Input: part model. Units: mm. Frame: model coordinates. A direction names the side the tool comes from. Coordinates: 2 decimals unless noted, no trailing zeros. Order: outer loops, then holes, each group sorted by start corner. A loop starts at its lowest first (then second) coordinate and runs counter-clockwise, first axis right, second up.
from build123d import *

# Parameters (mm, degrees)
F1_DEPTH     = 30
F2_R         = 14.99999
F4_DEPTH     = 219.001
F5_T1_DEPTH  = 2e-05
F5_T6_ANGLE  = 163.702935025
F5_T12_ANGLE = 163.702935025
F5_T18_ANGLE = 163.702935025
F5_T24_ANGLE = 163.702935025
F6_SIZE      = 5
F7_R         = 2.5
F8_DEPTH     = 139.001
F9_W         = 20
F9_H         = 20
F11_R        = 2.5
F12_DEPTH    = 20.001
F13_SIZE     = 2.5
F14_W        = 5
F14_H        = 25
F15_DEPTH    = 30
F16_R        = 14.99999
F17_R        = 5
F18_DEPTH    = 7.5
F19_SIZE     = 2.49999


# Not quite as in the source:
# - a fillet or chamfer that OpenCascade refuses, or shapes differently, is made with other operations: its cross-section is extruded or revolved along the edge and cut away or added
# - a fillet or chamfer is up to 0.001 mm smaller than in the source, because OpenCascade refuses the exact size


with BuildPart() as f1:
    # F0 (on Front) → F1 (new body)
    with BuildSketch(Plane.XZ):
        Polygon((-109.5, 0), (0, 0), (109.5, 0), (109.5, 20), (29.5, 20), (29.5, 50), (19.5, 50), (19.5, 20), (0, 20), (-19.5, 20), (-19.5, 50), (-29.5, 50), (-29.5, 20), (-109.5, 20), align=None)
    extrude(amount=F1_DEPTH)

    # F2 (radius 15 in the source; OpenCascade refuses exactly that, so slightly less here)
    f2_edges = [f1.edges().sort_by_distance(p)[0] for p in [
        (-69.5, 0, 20),
        (-69.5, -30, 20),
        (69.5, 0, 20),
        (69.5, -30, 20),
    ]]
    fillet(f2_edges, radius=F2_R)

    # F3 (on face) → F4 (cut, through all)
    with BuildSketch(Plane(origin=(-109.5, 0, 0), x_dir=(0, -1, 0), z_dir=(-1, 0, 0))):
        with BuildLine():
            Line((25, 0), (25, 5))
            ThreePointArc((25, 5), (15, 15), (5, 5))
            Line((5, 5), (5, 0))
            Line((5, 0), (25, 0))
        make_face()
    extrude(amount=-F4_DEPTH, mode=Mode.SUBTRACT)

    # F5: chamfer of 7.5 on 4 edges, made by hand

    # F5_s2 → F5_t1 (join)
    with BuildSketch(Plane.XZ.offset(14.99999)):
        Polygon((-37, 20), (-29.5, 27.5), (-29.5, 20), align=None)
        Polygon((37, 20), (29.5, 27.5), (29.5, 20), align=None)
    extrude(amount=F5_T1_DEPTH)


with BuildPart() as f5_tool4:
    # F5_s5 → F5_t6 (revolve)
    with BuildSketch(Plane(origin=(0, -12.4720838446, -3.6463990318), x_dir=(1, 0, 0), z_dir=(0, -0.9598196681, -0.2806175417))):
        Polygon((-37, -5.9916217418), (-29.5, -13.4916217418), (-29.5, -5.9916217418), align=None)
    revolve(axis=Axis((-29.5, -14.99999, 5.00001), (1, 0, 0)), revolution_arc=F5_T6_ANGLE)

    split(bisect_by=Plane.XZ, keep=Keep.TOP)

    split(bisect_by=Plane.XY, keep=Keep.TOP)


with BuildPart() as f1_1:
    add(f1.part)

    # F5_t3: union F5_tool4
    add(f5_tool4.part)


with BuildPart() as f5_tool10:
    # F5_s11 → F5_t12 (revolve)
    with BuildSketch(Plane(origin=(0, -12.4720838446, -3.6463990318), x_dir=(1, 0, 0), z_dir=(0, -0.9598196681, -0.2806175417))):
        Polygon((29.5, -13.4916217418), (37, -5.9916217418), (29.5, -5.9916217418), align=None)
    revolve(axis=Axis((29.5, -14.99999, 5.00001), (1, 0, 0)), revolution_arc=F5_T12_ANGLE)

    split(bisect_by=Plane.XZ, keep=Keep.TOP)

    split(bisect_by=Plane.XY, keep=Keep.TOP)


with BuildPart() as f1_2:
    add(f1_1.part)

    # F5_t9: union F5_tool10
    add(f5_tool10.part)


with BuildPart() as f5_tool16:
    # F5_s17 → F5_t18 (revolve)
    with BuildSketch(Plane.XZ.offset(15.00001)):
        Polygon((37, 20), (29.5, 27.5), (29.5, 20), align=None)
    revolve(axis=Axis((29.5, -15.00001, 5.00001), (1, 0, 0)), revolution_arc=F5_T18_ANGLE)

    split(bisect_by=Plane.XY, keep=Keep.TOP)

    split(bisect_by=Plane.XZ.offset(30), keep=Keep.BOTTOM)


with BuildPart() as f1_3:
    add(f1_2.part)

    # F5_t15: union F5_tool16
    add(f5_tool16.part)


with BuildPart() as f5_tool22:
    # F5_s23 → F5_t24 (revolve)
    with BuildSketch(Plane.XZ.offset(15.00001)):
        Polygon((-37, 20), (-29.5, 27.5), (-29.5, 20), align=None)
    revolve(axis=Axis((-29.5, -15.00001, 5.00001), (1, 0, 0)), revolution_arc=F5_T24_ANGLE)

    split(bisect_by=Plane.XY, keep=Keep.TOP)

    split(bisect_by=Plane.XZ.offset(30), keep=Keep.BOTTOM)


with BuildPart() as f1_4:
    add(f1_3.part)

    # F5_t21: union F5_tool22
    add(f5_tool22.part)

    # F6
    f6_edges = [f1_4.edges().sort_by_distance(p)[0] for p in [
        (-24.5, 0, 50),
        (-24.5, -30, 50),
        (24.5, 0, 50),
        (24.5, -30, 50),
    ]]
    chamfer(f6_edges, length=F6_SIZE)

    # F7 (on face) → F8 (cut, through all)
    with BuildSketch(Plane.YZ.offset(29.5)):
        with Locations((-15, 40)):
            Circle(F7_R)
    extrude(amount=-F8_DEPTH, mode=Mode.SUBTRACT)

    # F9 (on face) → F10 (join, up to the next surface of F1)
    with BuildSketch(Plane(origin=(0, 0, 0), x_dir=(1, 0, 0), z_dir=(0, 0, -1))):
        with Locations((0, 15)):
            Rectangle(F9_W, F9_H)
    extrude(until=Until.NEXT, dir=(0, 0, 1))

    # F11 (on face) → F12 (cut, through all)
    with BuildSketch(Plane.XY.offset(20)):
        with Locations((0, -15)):
            Circle(F11_R)
    extrude(amount=-F12_DEPTH, mode=Mode.SUBTRACT)

    # F13
    f13_edges = [f1_4.edges().sort_by_distance(p)[0] for p in [
        (-29.5, -17.5, 40),
        (29.5, -17.5, 40),
    ]]
    chamfer(f13_edges, length=F13_SIZE)

    # F14 (on face) → F15 (join, through all)
    with BuildSketch(Plane.XZ.offset(30)):
        with Locations((-112, 12.5)):
            Rectangle(F14_W, F14_H)
        with Locations((112, 12.5)):
            Rectangle(F14_W, F14_H)
    extrude(amount=-F15_DEPTH)

    # F16 (radius 15 in the source; OpenCascade refuses exactly that, so slightly less here)
    f16_edges = [f1_4.edges().sort_by_distance(p)[0] for p in [
        (112, 0, 25),
        (112, -30, 25),
        (-112, -30, 25),
        (-112, 0, 25),
    ]]
    fillet(f16_edges, radius=F16_R)

    # F17 (on face) → F18 (cut)
    with BuildSketch(Plane(origin=(0, 0, 0), x_dir=(1, 0, 0), z_dir=(0, 0, -1))):
        with Locations((0, 15)):
            Circle(F17_R)
    extrude(amount=-F18_DEPTH, mode=Mode.SUBTRACT)

    # F19 (size 2.5 in the source; OpenCascade refuses exactly that, so slightly less here)
    f19_edges = [f1_4.edges().sort_by_distance(p)[0] for p in [
        (-2.5, -15, 7.5),
    ]]
    chamfer(f19_edges, length=F19_SIZE)


solid = f1_4.part
Item 1: Draft query along Z for faces 6 (the face through (-23.2, -15.54, 37.56)), 7 (the face through (72.74, -25.49, 15.72)), 8 (the face through (-27.12, -15.57, 37.44)), 9 (the face through (-0.346, -12.366, 9.844)). Return one class per face: pulls with the +Z half, pulls with the -Z half, needs draft (parallel to the pull), parting line crosses it, or undercut.
Response values:
face 6: undercut
face 7: pulls with the +Z half
face 8: undercut
face 9: pulls with the -Z half
Item 2: Cut plane D-D on z = 12. Count the separate pieces of the cut face and the enclosed holes in it, then the cut area to 3 significant figures.
Response values:
separate pieces: 1
enclosed holes: 3
area: 3,500 mm2
Item 3: Pin query (flat end, axial travel): pin 1 Ø5 at (y, z) = (-7.5, 34) entering from +X; pin 2 Ø2 at (y, z) = (-4.5, 31) entering from -X; pin 3 Ø6 at (x, y) = (-91.5, -9.5) entering from -Z; pin 4 Ø3 at (x, y) = (0, -15) entering from -Z. Return the tip coordinate at first contact, or that it passes through.
Response values:
pin 1: stops at x = 29.5
pin 2: stops at x = -29.5
pin 3: stops at z = 10.27
pin 4: passes through
Item 4: Cut plane B-B on z = 40. Return loops of the section in (x, y), then the cut area to 4 significant figures.
Response values:
outline: (-29.5, -30) - (-19.5, -30) - (-19.5, -17.5) - (-27, -17.5) - (-29.5, -20) - close; (-29.5, -10) - (-27, -12.5) - (-19.5, -12.5) - (-19.5, 0) - (-29.5, 0) - close; (19.5, -30) - (29.5, -30) - (29.5, -20) - (27, -17.5) - (19.5, -17.5) - close; (19.5, -12.5) - (27, -12.5) - (29.5, -10) - (29.5, 0) - (19.5, 0) - close
area: 487.5 mm2
Item 5: Ray query, probe 1 along X at (y, z) = (-15, 3.25); probe 2 along X at (y, z) = (-9.5, 38); probe 3 along Y at (x, z) = (0, 3.25). Return the intervals inside material, ascending.
Response values:
probe 1: x = -114.5 to -109.5, -10 to -5, 5 to 10, 109.5 to 114.5
probe 2: x = -29.5 to -19.5, 19.5 to 29.5
probe 3: y = -30 to -20, -10 to 0
Item 6: Access query for faces 1 (the face through (-111.96, -25.72, 20.49)), 2 (the face through (0, -11, 20)), 3 (the face through (-60, -25, 2)), 4 (the face through (-73.76, -4.51, 15.72)), 5 (the face through (112.04, -4.28, 20.49)). Directions: +Z, -Z, +X, -X, +Y, -Y. A direction counts if a zero-diameter tool reaches every point of the face in a straight line with its end or side. Return the directions, or none.
Response values:
face 1: +Z, -X, -Y
face 2: +Z, +Y, -Y
face 3: -Z
face 4: +Z, +Y
face 5: +Z, +X, +Y
